```python
from build123d import *

# Parameters (mm, degrees)
F0_W     = 50
F0_H     = 50
F1_DEPTH = 20
F2_R     = 10
F3_DEPTH = 25
F4_SIZE  = 5


with BuildPart() as f1:
    # F0 (on Top) → F1 (new body)
    with BuildSketch(Plane.XY):
        with Locations((25, 25)):
            Rectangle(F0_W, F0_H)
    extrude(amount=F1_DEPTH)

    # F2 (on face) → F3 (cut)
    with BuildSketch(Plane.XY.offset(20)):
        with Locations((24.133066, 27.181452)):
            Circle(F2_R)
    extrude(amount=-F3_DEPTH, mode=Mode.SUBTRACT)

    # F4
    f4_edges = [f1.edges().sort_by_distance(p)[0] for p in [
        (14.133066, 27.181452, 20),
        (14.133066, 27.181452, 0),
    ]]
    chamfer(f4_edges, length=F4_SIZE)


solid = f1.part
```
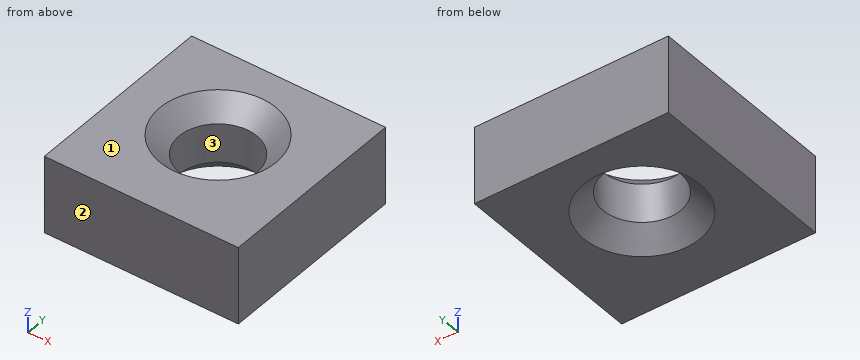
Could you check a few things on this model? Use its own coordinates, in mm. Face numbers are marked on the shaded views. Coordinates: 2 decimals unless noted, no trailing zeros. Write each loop counter-clockwise with the first axis right and the second up, starting at its lowest first coordinate (ties: lowest second). Pieces come first, ordered by that corner, then holes. Notation, with made-up numbers: M -7,62 L 34,62 A3 ccw 34,67 Z; hole C -31.75,-32 d5. An arc over 180 degrees is marked long. Answer as CSV lines item,"result". Start each with the question number.
1) I want a section at A-A, the plane z = 3. Please give me the cut outline in (x, y), and give its area (3 significant figures).
2) We'd pull the mould along Y, two halves only. Please class the marked faces 1, 2 and 3: +Y half, -Y half, draft (parallel to the pull), parting line (faces both ways), or undercut.
3) For P1, Ø12, axis at x = 21.5, y = 32, coming from the +Z side, with a flat end and sliding along its axis, tell me the tip position at first contact or that it passes through.
4) Please list where these lines run through material, in increasing order: line 1 (Y direction, x = 32.5, z = 14.5); line 2 (X direction, y = 34, z = 3.75); line 3 (Y direction, x = 21, z = 14.25). Write a range as from..to.
5) I want a section at B-B, the plane z = 18.75. Please give me the cut outline in (x, y).
Data:
1,outline,"M 0,0 L 50,0 L 50,50 L 0,50 Z; hole C 24.13,27.18 d24"
1,area,"2,050 mm^2"
2,face 1,"draft"
2,face 2,"-Y half"
2,face 3,"undercut"
3,P1,"stops at z = 16.49"
4,line 1,"y = 0..21.7, 32.66..50"
4,line 2,"x = 0..15.18, 33.08..50"
4,line 3,"y = 0..17.68, 36.68..50"
5,outline,"M 0,0 L 50,0 L 50,50 L 0,50 Z; hole C 24.13,27.18 d27.5"
